Design review of the part built by this model. Coordinates are the model's own, in mm. A direction names the side the tool comes from. Round coordinates to 2 decimals unless told otherwise and drop trailing zeros. Write each loop counter-clockwise with the first axis right and the second up, starting at its lowest first coordinate (ties: lowest second). Pieces come first, ordered by that corner, then holes. Notation, with made-up numbers: (45.5, 80.5) -> (81.5, 80.5) arc R13 ccw to (81.5, 97.5) -> close; hole circle Ø5 at (-0.5, -27.5). An arc over 180 degrees is marked (long way). Write item = value, one per line. Start each with the question number.
Item 1: To check wall thickness, follow L1, parallel to X at y = -0.25, z = -29; L2, parallel to Z at x = 4.5, y = -11.5; L3, parallel to Z at x = -10, y = -11.25. State the ranges of each line that lie inside material, in increasing order.
Item 2: Add section C-C, the plane y = 1.25. State how many separate pieces and enclosed holes the cut face has, then the cut area to 3 significant figures.
Item 3: For pin 1 Ø1.3 at (x, y) = (30.5, -5) entering from +Z; pin 2 Ø1.4 at (y, z) = (-6.5, 43.5) entering from +X; pin 3 Ø2.5 at (y, z) = (-1, 48) entering from +X, all flat-tipped, find the tip position at first contact; note any pin that passes through.
Item 4: Mouldability with a two-part tool opening along X and no side actions: class faces 4 (the flat face through (-31, 0, -35)), 5 (the flat face through (-1, 0, -45)), 6 (the flat face through (45, 0, -1)) as released by +X, released by -X, zero draft, split by the parting line, or undercut.
Item 5: Add section B-B, the plane z = -5.5. State the section outline as (x, y) points, then the cut area to 3 significant figures.
Item 6: Add section A-A, the plane x = -13. State the section outline as (y, z) points, then the cut area to 3 significant figures.
Item 7: Machinability: for faces 1 (the flat face through (0, 7, 40.213)), 2 (the flat face through (-31, 0, 35)), 3 (the flat face through (5.222, 0, 47)), which of the approach directions +Z, -Z, +X, -X, +Y, -Y give a long, thin tool a straight path to every point of the face, cutting with its end or side? Answer none if there is none.
Item 8: Add section D-D, the plane x = -23. State the section outline as (y, z) points.
from build123d import *

# Parameters (mm, degrees)
F0_W     = 5.222296
F0_H     = 4.786847
F1_DEPTH = 2.5
F2_DEPTH = 12.5


with BuildPart() as f1:
    # F0 (on Front) → F1 (new body, symmetric)
    with BuildSketch(Plane.XZ):
        with Locations((2.611148, 47.393423)):
            Rectangle(F0_W, F0_H)
        with Locations((-2.611148, 47.393423)):
            Rectangle(F0_W, F0_H)
        Polygon((0, 45), (-5.222296, 45), (-5.222296, 40.213153), (5.222296, 40.213153), (5.222296, 45), align=None)
    extrude(amount=F1_DEPTH, both=True)

    # F0 (on Front) → F2 (join, symmetric)
    with BuildSketch(Plane.XZ):
        with BuildLine():
            Line((-5.222296, 45), (-40, 45))
            ThreePointArc((-40, 45), (-43.535534, 43.535534), (-45, 40))
            Line((-45, 40), (-45, -40))
            ThreePointArc((-45, -40), (-43.535534, -43.535534), (-40, -45))
            Line((-40, -45), (40, -45))
            ThreePointArc((40, -45), (43.535534, -43.535534), (45, -40))
            Line((45, -40), (45, 40))
            ThreePointArc((45, 40), (43.535534, 43.535534), (40, 45))
            Line((40, 45), (5.222296, 45))
            Line((5.222296, 45), (5.222296, 40.213153))
            Line((5.222296, 40.213153), (-5.222296, 40.213153))
            Line((-5.222296, 40.213153), (-5.222296, 45))
        make_face()
        with BuildLine():
            Line((3.352741, 35), (8.352741, 35))
            Line((8.352741, 35), (15, 35))
            Line((15, 35), (27.810507, 35))
            Line((27.810507, 35), (30.06182, 35))
            Line((30.06182, 35), (32.644888, 35))
            ThreePointArc((32.644888, 35), (34.236806, 34.340606), (34.8962, 32.748687))
            Line((34.8962, 32.748687), (34.8962, -32.748687))
            ThreePointArc((34.8962, -32.748687), (34.236806, -34.340606), (32.644888, -35))
            Line((32.644888, -35), (30.06182, -35))
            Line((30.06182, -35), (27.810507, -35))
            Line((27.810507, -35), (15, -35))
            Line((15, -35), (8.352741, -35))
            Line((8.352741, -35), (3.352741, -35))
            Line((3.352741, -35), (0, -35))
            Line((0, -35), (-3.352741, -35))
            Line((-3.352741, -35), (-8.352741, -35))
            Line((-8.352741, -35), (-15, -35))
            Line((-15, -35), (-27.810507, -35))
            Line((-27.810507, -35), (-30.06182, -35))
            Line((-30.06182, -35), (-32.701636, -35))
            ThreePointArc((-32.701636, -35), (-34.293555, -34.340606), (-34.952949, -32.748687))
            Line((-34.952949, -32.748687), (-34.952949, 32.748687))
            ThreePointArc((-34.952949, 32.748687), (-34.293555, 34.340606), (-32.701636, 35))
            Line((-32.701636, 35), (-30.06182, 35))
            Line((-30.06182, 35), (-27.810507, 35))
            Line((-27.810507, 35), (-15, 35))
            Line((-15, 35), (-8.352741, 35))
            Line((-8.352741, 35), (-3.352741, 35))
            Line((-3.352741, 35), (0, 35))
            Line((0, 35), (3.352741, 35))
        make_face(mode=Mode.SUBTRACT)
        with BuildLine():
            ThreePointArc((-20, 30), (-18.535534, 33.535534), (-15, 35))
            Line((-15, 35), (-27.810507, 35))
            Line((-27.810507, 35), (-30.06182, 35))
            ThreePointArc((-30.06182, 35), (-28.469901, 34.340606), (-27.810507, 32.748687))
            Line((-27.810507, 32.748687), (-27.810507, -32.748687))
            ThreePointArc((-27.810507, -32.748687), (-28.469901, -34.340606), (-30.06182, -35))
            Line((-30.06182, -35), (-27.810507, -35))
            Line((-27.810507, -35), (-15, -35))
            ThreePointArc((-15, -35), (-18.535534, -33.535534), (-20, -30))
            Line((-20, -30), (-20, 30))
        make_face()
        with BuildLine():
            Line((27.810507, 35), (15, 35))
            ThreePointArc((15, 35), (18.535534, 33.535534), (20, 30))
            Line((20, 30), (20, -30))
            ThreePointArc((20, -30), (18.535534, -33.535534), (15, -35))
            Line((15, -35), (27.810507, -35))
            Line((27.810507, -35), (30.06182, -35))
            ThreePointArc((30.06182, -35), (28.469901, -34.340606), (27.810507, -32.748687))
            Line((27.810507, -32.748687), (27.810507, 32.748687))
            ThreePointArc((27.810507, 32.748687), (28.469901, 34.340606), (30.06182, 35))
            Line((30.06182, 35), (27.810507, 35))
        make_face()
    extrude(amount=F2_DEPTH, both=True)


solid = f1.part
Result set:
q1.L1 = -45 to -34.95, -27.81 to -20, 20 to 27.81, 34.9 to 45
q1.L2 = -45 to -35, 35 to 40.21
q1.L3 = -45 to -35, 35 to 45
q2.separate_pieces = 1
q2.enclosed_holes = 3
q2.area = 4,360 mm²
q3.pin_1 = 45
q3.pin_2 = 44.14
q3.pin_3 = 5.22
q4.face_4 = undercut
q4.face_5 = zero draft
q4.face_6 = released by +X
q5.outline = (-45, -12.5) -> (-34.95, -12.5) -> (-34.95, 12.5) -> (-45, 12.5) -> close; (-27.81, -12.5) -> (-20, -12.5) -> (-20, 12.5) -> (-27.81, 12.5) -> close; (20, -12.5) -> (27.81, -12.5) -> (27.81, 12.5) -> (20, 12.5) -> close; (34.9, -12.5) -> (45, -12.5) -> (45, 12.5) -> (34.9, 12.5) -> close
q5.area = 894 mm²
q6.outline = (-12.5, -45) -> (12.5, -45) -> (12.5, -35) -> (-12.5, -35) -> close; (-12.5, 35) -> (12.5, 35) -> (12.5, 45) -> (-12.5, 45) -> close
q6.area = 500 mm²
q7.face_1 = +Z, +Y
q7.face_2 = +Y, -Y
q7.face_3 = +Z, +X, +Y, -Y
q8.outline = (-12.5, -45) -> (12.5, -45) -> (12.5, 45) -> (-12.5, 45) -> close
